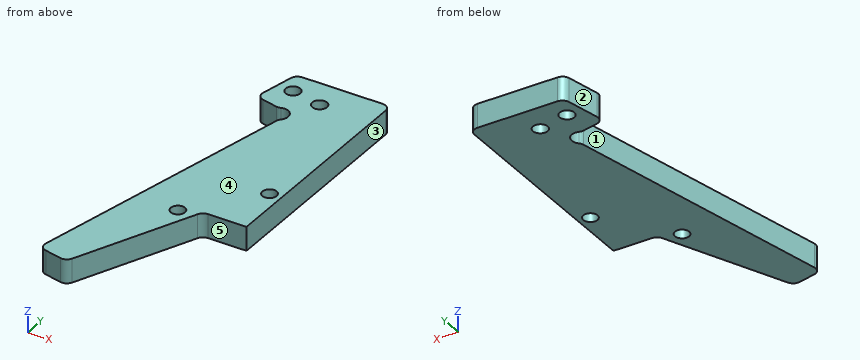
Autodesk Inventor part; units mm, degrees
ref_plane "YZ Plane" through (0, 0, 0) normal (1, 0, 0) x (0, 1, 0)
ref_plane "XZ Plane" through (0, 0, 0) normal (0, 1, 0) x (-1, 0, 0)
ref_plane "XY Plane" through (0, 0, 0) normal (0, 0, 1) x (1, 0, 0)
sketch "Sketch1" plane through (0, 0, 0) normal (0, 0, 1) x (1, 0, 0)
  line L0 (0, 0) -> (0, 136.525) construction
  line L1 (-11.7886, 12.2907) -> (-39.6863, 18.4755) construction
  line L2 (-39.6863, 18.4755) -> (-33.3297, 47.1481) construction
  line L3 (-33.3297, 47.1481) -> (-5.432, 40.9633)
  line L4 (-5.432, 40.9633) -> (-11.7886, 12.2907) construction
  line L5 (-39.6863, 18.4755) -> (-5.432, 40.9633) construction
  line L6 (-33.3297, 47.1481) -> (-11.7886, 12.2907) construction
  circle A0 centre (-53.975, 12.7) radius 3.175 construction
  circle A1 centre (-53.975, 12.7) radius 6.35 construction
  line L7 (0, 0) -> (-54.712, 6.3929) construction
  line L8 (-59.6703, 15.5082) -> (0, 136.525) construction
  line L9 (-27.1302, 45.7737) -> (-37.4529, 28.5497) construction
  line L10 (-11.6315, 42.3377) -> (-9.5552, 22.3649) construction
  line L11 (-19.3809, 44.0557) -> (-25.7374, 15.3831) construction
  line L12 (0, 92.075) -> (-19.7574, 96.4551) construction
  line L13 (-35.3766, 8.5768) -> (-19.8779, 5.1408) construction
  line L14 (-19.8779, 5.1408) -> (-21.2523, -1.0586) construction
  line L15 (-21.2523, -1.0586) -> (-36.751, 2.3773) construction
  line L16 (-36.751, 2.3773) -> (-35.3766, 8.5768) construction
  line L17 (-35.3766, 8.5768) -> (-41.27, 4.8223) construction
  line L18 (-19.8779, 5.1408) -> (-17.9381, 2.096) construction
  line L19 (-5.432, 40.9633) -> (-33.3297, 47.1481) construction
  line L20 (-33.3297, 47.1481) -> (-32.2475, 52.0296) construction
  line L21 (-32.2475, 52.0296) -> (-4.3498, 45.8448) construction
  line L22 (-4.3498, 45.8448) -> (-5.432, 40.9633) construction
  line L23 (-53.2878, 15.7997) -> (-53.975, 12.7) construction
  line L24 (-53.975, 12.7) -> (-57.0747, 13.3872) construction
  line L25 (-27.6272, 6.8588) -> (-34.4992, -24.1386) construction
  line L26 (-31.8676, 50.076) -> (-5.5198, 44.2349)
  line L27 (-5.5198, 44.2349) -> (-4.489, 48.8845) construction
  line L28 (-4.489, 48.8845) -> (-30.8368, 54.7256) construction
  line L29 (-30.8368, 54.7256) -> (-31.8676, 50.076) construction
  line L30 (-31.3522, 52.4008) -> (-5.0044, 46.5597) construction
  circle A2 centre (-29.0274, 51.8854) radius 1.4732 construction
  circle A3 centre (-22.8279, 50.5111) radius 1.4732 construction
  circle A4 centre (-16.6284, 49.1367) radius 1.4732
  circle A5 centre (-10.4289, 47.7623) radius 1.4732
  circle A6 centre (-10.3614, 84.7398) radius 1.4732 construction
  line L31 (-53.975, 12.7) -> (-13.3751, 95.0402) construction
  line L32 (-32.2923, 56.6744) -> (0, 49.5153)
  circle A7 centre (-10.3614, 84.7398) radius 4.7625 construction
  line L33 (-4.7625, 50.5712) -> (-4.7625, 93.1308) construction
  line L34 (-27.5056, 55.6132) -> (-14.3936, 82.2055) construction
  line L35 (-5.6003, 84.6261) -> (-4.7625, 84.4403) construction
  line L36 (-17.9381, 2.096) -> (0, 2.096) construction
  line L37 (0, 2.096) -> (0, -1.079) construction
  line L38 (0, -1.079) -> (-17.9381, -1.079) construction
  line L39 (-17.9381, -1.079) -> (-17.9381, 2.096) construction
  circle A8 centre (-12.7, 7.9375) radius 1.5875 construction
  line L40 (-12.7, 7.9375) -> (0, 7.9375)
  line L41 (0, 7.9375) -> (-17.9381, 2.096) construction
  circle A9 centre (-12.7, 7.9375) radius 3.175 construction
  line L42 (-9.525, 7.9375) -> (-9.525, 4.8357) construction
  line L43 (-9.525, 7.9375) -> (0, 7.9375) construction
  line L44 (-17.9187, 46.9837) -> (-16.8879, 51.6333)
  line L45 (-12.4942, 45.7811) -> (-26.2381, -16.2137)
  line L46 (0, 66.675) -> (0, 7.9375)
  line L47 (-26.2381, -16.2137) -> (-20.0386, -17.5881)
  line L48 (-20.0386, -17.5881) -> (-8.7313, 7.9375)
  circle A10 centre (-12.7, 6.35) radius 1.4224
  line L49 (0, 13.4938) -> (-4.7625, 13.4938) construction
  line L50 (-4.7625, 13.4938) -> (-4.7625, 24.6063) construction
  line L51 (-4.7625, 24.6063) -> (0, 24.6063) construction
  line L52 (0, 24.6063) -> (0, 13.4938)
  line L53 (-4.7625, 19.05) -> (0, 19.05) construction
  circle A11 centre (-2.3813, 19.05) radius 1.4224
  line L54 (-20.7405, 8.5842) -> (-9.7454, 58.18)
  line L55 (-9.7454, 58.18) -> (-3.5459, 56.8056) construction
  line L56 (-3.5459, 56.8056) -> (-14.5411, 7.2098) construction
  line L57 (-14.5411, 7.2098) -> (-20.7405, 8.5842)
  line L58 (-12.7, 6.35) -> (-12.7, 7.9375) construction
  line L59 (-11.5442, 1.5875) -> (-9.525, 1.5875)
  line L60 (-9.525, 1.5875) -> (-9.525, 7.9375)
  line L61 (-9.525, 7.9375) -> (-11.5442, 7.9375)
  line L62 (-11.5442, 7.9375) -> (-11.5442, 1.5875) construction
  line L63 (-9.7454, 58.18) -> (-15.9449, 59.5544)
  line L64 (-15.9449, 59.5544) -> (-14.6504, 65.3933)
  line L65 (-14.6504, 65.3933) -> (0, 66.675)
  line L66 (-9.7454, 58.18) -> (-17.3193, 53.3549) construction
  arc A12 (-10.2313, 55.9882) -> (-11.9373, 58.6659) centre (-11.0843, 57.3271) ccw
  line L67 (-4.7625, 57.15) -> (0, 57.15) construction
  circle A13 centre (-2.3813, 57.15) radius 1.4224
  circle A14 centre (-2.3813, 63.5) radius 1.4224
  line L68 (-20.9307, 44.3993) -> (-18.8691, 53.6985)
  line L69 (-12.4942, 45.7811) -> (-16.2811, 43.3685) construction
  arc A15 (-13.0773, 43.1508) -> (-15.1244, 46.3642) centre (-14.1008, 44.7575) ccw
  line L70 (-18.8691, 53.6985) -> (0, 53.6985)
  line L71 (-13.1814, 42.6813) -> (-14.788, 41.6578) construction
  circle A16 centre (-14.788, 41.6578) radius 1.905
  point P0 (-22.5591, 29.7194)
  point P1 (-20.4869, 2.3938)
  point P2 (-36.3367, 4.2458)
  point P3 (-51.1668, 18.3953)
  point P4 (-11.1125, 7.9375)
  point P5 (-11.4283, 6.9872)
  point P6 (-11.9574, 7.9375)
  point P7 (-13.9717, 6.9872)
  point P8 (-9.525, 6.1457)
  point P9 (-15.8116, 43.2644)
  point P10 (-13.7645, 40.0511)
  dimension "d74" = 6.35
  dimension "d122" = 3.81
  dimension "d13" = 136.525
  dimension "d14" = 29.3687
  dimension "d15" = 28.575
  dimension "d16" = 12.5
  dimension "d17" = 6.35
  dimension "d19" = 53.975
  dimension "d22" = 12.7
  dimension "d23" = 7.9375
  dimension "d24" = 19.05
  dimension "d26" = 102.5
  dimension "d29" = 6.35
  dimension "d31" = 7.9375
  dimension "d34" = 5
  dimension "d35" = 26.9875
  dimension "d38" = 31.75
  dimension "d40" = 26.9875
  dimension "d41" = 4.7625
  dimension "d42" = 2.9464
  dimension "d43" = 2.3813
  dimension "d46" = 6.35
  dimension "d51" = 2.9464
  dimension "d52" = 79.7719
  dimension "d53" = 6.35
  dimension "d54" = 9.525
  dimension "d55" = 4.7625
  dimension "d56" = 4.7625
  dimension "d60" = 12.7
  dimension "d61" = 3.175
  dimension "d63" = 3.175
  dimension "d66" = 3.175
  dimension "d67" = 12.7
  dimension "d72" = 8.7312
  dimension "d73" = 7.9375
  dimension "d75" = 34.925
  dimension "d80" = 12.7
  dimension "d82" = 7.9375
  dimension "d83" = 63.5
  dimension "d84" = 66.675
  dimension "d85" = 6.35
  dimension "d86" = 92.075
  dimension "d87" = 2.8448
  dimension "d88" = 4.7625
  dimension "d89" = 11.1125
  dimension "d90" = 2.8448
  dimension "d91" = 19.05
  dimension "d92" = 6.35
  dimension "d93" = 50.8
  dimension "d94" = 25.4
  dimension "d95" = 8.7312
  dimension "d96" = 9.525
  dimension "d97" = 6.35
  dimension "d99" = 6.35
  dimension "d101" = 3.175
  dimension "d106" = 2.8448
  dimension "d107" = 57.15
  dimension "d110" = 6.35
  dimension "d119" = 85
  dimension "d120" = 3.175
  dimension "d121" = 3.81
extrude "Extrusion1" add sketch "Sketch1" along normal blind 4.7625 contours L68 L26 L45 A16 L3 | L68 L32 L54 A15 L26 | L45 A15 L54 L32 L46 L40 L60 L48 L47 A16 | L70 L54 L32 | L45 A15 | A15 L26 | L54 L70 L46 L32 | L60 L40 L48
fillet "Fillet1" radius 1.5875 3 edges at (-26.2381, -16.2137, 2.3813) (-20.0386, -17.5881, 2.3813) (-8.7313, 7.9375, 2.3813)
fillet "Fillet4" radius 1.5875 5 edges at (-18.8691, 53.6985, 2.3813) (0, 53.6985, 2.3813) (-20.9307, 44.3993, 2.3813) (-15.8116, 43.2644, 2.3813) (-13.7645, 40.0511, 2.3813)
equation "\"d56\" = d55"
properties part number "Uprights" material "UHMW, White"
Can you work these out from the model? Positions are in its coordinate system, mm. Face numbers are marked on the shaded views. A direction names the side the tool comes from. Coordinates: 2 decimals unless noted, no trailing zeros. Write each loop counter-clockwise with the first axis right and the second up, starting at its lowest first coordinate (ties: lowest second). Pieces come first, ordered by that corner, then holes. Notation, with made-up numbers: M -25,24 L -3,24 A10 cw -3,28 Z; hole C 31,3 d4. An arc over 180 degrees is marked long. Write item = value, one per line. Start each with the question number.
Q1. If we section it at D-D, the plane y = 31: Write out the boundary of the cut face in (x, z).
Q2. On a 3-axis mill with a long thin cutter (end or side, diameter ignored), from which of +Z, -Z, +X, -X, +Y, -Y can I reach the whole of each face in a straight line? I mean the marked faces 4 and 5. Say none if no direction works.
Q3. If we section it at B-B, the plane x = -3: Write out the boundary of the cut face in (y, z).
Q4. If I drill on L1, parallel to Y at x = -6.75, z = 2.55; L2, parallel to Y at x = -12.7, z = 1.95; L3, parallel to X at y = 18, z = 0.8, over which ranges is the centre line in solid material (lowest first)? Write a range as [from, to].
Q5. If we section it at C-C, the plane z = 2.35: State how many separate pieces and enclosed holes the cut face has, then the cut area to 3 significant figures.
Q6. I'm going to push flat-ended pins straight in: pin 1 (1 mm diameter, centred on x = -13, z = 4, fed in from -Y); pin 2 (2 mm diameter, centred on x = -22.5, z = 3, fed in from -Y). Where does each tip first touch, or does it pass through?
Q7. Thinking about a two-plate mould opening in Y: for the marked faces 1, 2 and 3, which applies, released by +Y, released by -Y, zero draft, split by the parting line, or undercut?
Q8. If we section it at A-A, the plane y = 19.05: Write out the boundary of the cut face in (x, z), then the cut area to 3 significant figures.
Check sheet entries:
q1.outline = M -15.77,0 L 0,0 L 0,4.76 L -15.77,4.76 Z
q2.face_4 = +Z, +X, -X, +Y, -Y
q2.face_5 = +Z, -Z, +X, -Y
q3.outline = M 7.94,0 L 17.77,0 L 17.77,4.76 L 7.94,4.76 Z; M 20.33,0 L 53.7,0 L 53.7,4.76 L 20.33,4.76 Z
q4.L1 = [7.94, 53.7]
q4.L2 = [-1.02, 4.93], [7.77, 53.7]
q4.L3 = [-18.65, -3.34], [-1.42, 0]
q5.separate_pieces = 1
q5.enclosed_holes = 4
q5.area = 1,010 mm²
q6.pin_1 = -2.83
q6.pin_2 = -17.26
q7.face_1 = undercut
q7.face_2 = released by +Y
q7.face_3 = zero draft
q8.outline = M -18.42,0 L -3.8,0 L -3.8,4.76 L -18.42,4.76 Z; M -0.96,0 L 0,0 L 0,4.76 L -0.96,4.76 Z
q8.area = 74.2 mm²
